from build123d import *

# Parameters (mm, degrees)
SKETCH_1_R          = 7.5
SKETCH_1_R_2        = 7
EXTRUDE_1_DEPTH     = 200
EXTRUDE_START       = -1
SKETCH_2_R          = 7
EXTRUDE_2_DEPTH     = 1
SKETCH_3_R          = 2.1
CUT_EXTRUDE_1_DEPTH = 10


with BuildPart() as part:
    # 草图1 → 凸台-拉伸1 (new body)
    with BuildSketch(Plane(origin=(0, 0, 0), x_dir=(1, 0, 0), z_dir=(0, 1, 0))):
        with Locations(Location((0, 0, 0), (0, 0, 270))):
            Circle(SKETCH_1_R)
        with Locations(Location((0, 0, 0), (0, 0, 270))):
            Circle(SKETCH_1_R_2, mode=Mode.SUBTRACT)
    extrude(amount=EXTRUDE_1_DEPTH)

    # 草图2 → 凸台-拉伸2 (add)
    with BuildSketch(Plane(origin=(0, 200, 0), x_dir=(1, 0, 0), z_dir=(0, 1, 0)).offset(EXTRUDE_START)):
        with Locations(Location((0, 0, 0), (0, 0, 270))):
            Circle(SKETCH_2_R)
    extrude(amount=EXTRUDE_2_DEPTH)

    # 草图3 → 切除-拉伸1 (cut)
    with BuildSketch(Plane(origin=(0, 200, 0), x_dir=(1, 0, 0), z_dir=(0, 1, 0))):
        with Locations(Location((0, 0, 0), (0, 0, 270))):
            Circle(SKETCH_3_R)
    extrude(amount=-CUT_EXTRUDE_1_DEPTH, mode=Mode.SUBTRACT)


solid = part.part
The listing builds one solid part. Answer for the finished solid, in the listing's coordinates (mm). A direction names the side the tool comes from. Round coordinates to 2 decimals unless told otherwise and drop trailing zeros. Write each loop counter-clockwise with the first axis right and the second up, starting at its lowest first coordinate (ties: lowest second). Pieces come first, ordered by that corner, then holes. Notation, with made-up numbers: M 27,53 L 69,53 A23 cw 69,87 Z; hole C 54,75 d1. An arc over 180 degrees is marked long. Write each question's results on one line, items separated by ' | '. Start each with the question number.
Item 1: A cutting plane is placed at C-C on y = 115.5. Write down the section's boundary in (x, z), and give its area (3 significant figures).
Item 2: For faces 1 (the face through (-2, 200, 2)), 2 (the face through (1.7, 199, 1.5)), determine the directions among +Z, -Z, +X, -X, +Y, -Y from which every point of the face is accessible in a straight line to the end or side of a thin tool.
Item 3: A cutting plane is placed at A-A on x = 0. Write down the section's boundary in (y, z).
Item 4: A cutting plane is placed at B-B on z = 0. Write down the section's boundary in (x, y).
Item 5: For a pull along Z with two mould halves and no side action, classify faces 3 (the face through (0.33, 98.6, -7.493)), 4 (the face through (-6.834, 98.107, -1.517)), 5 (the face through (-7, 0, -2)) as pulls with the +Z half, pulls with the -Z half, needs draft (parallel to the pull), parting line crosses it, or undercut.
Item 6: Straight lines are drawn through the part: L1, parallel to X at y = 55, z = 0; L2, parallel to Z at x = -2, y = 34; L3, parallel to Z at x = 1.5, y = 79. For each, find the intervals that lie inside material, in ascending order. Write a range as [from, to].
Item 7: Flat-ended cylindrical pins translate along their axes: pin 1 Ø5.5 at (x, z) = (0, 0) entering from -Y; pin 2 Ø1.5 at (x, y) = (1, 119.5) entering from -Z; pin 3 Ø1.5 at (x, y) = (1, 138) entering from +Z. Find the tip coordinate at first contact, or state that the pin passes through.
Check sheet entries:
1) outline: C 0,0 d15; hole C 0,0 d14 | area: 22.8 mm²
2) face 1: +Z, -Z, +X, -X, +Y | face 2: -Y
3) outline: M 0,-7.5 L 200,-7.5 L 200,-2.1 L 199,-2.1 L 199,-7 L 0,-7 Z; M 0,7 L 199,7 L 199,2.1 L 200,2.1 L 200,7.5 L 0,7.5 Z
4) outline: M -7.5,0 L -7,0 L -7,199 L -2.1,199 L -2.1,200 L -7.5,200 Z; M 2.1,199 L 7,199 L 7,0 L 7.5,0 L 7.5,200 L 2.1,200 Z
5) face 3: parting line crosses it | face 4: undercut | face 5: needs draft
6) L1: [-7.5, -7], [7, 7.5] | L2: [-7.23, -6.71], [6.71, 7.23] | L3: [-7.35, -6.84], [6.84, 7.35]
7) pin 1: y = 199 | pin 2: z = -7.5 | pin 3: z = 7.5
